Check sheet for the modelled part. Datum: model origin and axes. Units: mm. Face numbers are marked on the shaded views. Round coordinates to 2 decimals unless told otherwise and drop trailing zeros. Loops run counter-clockwise (first coordinate to the right, second up) from the corner with the lowest first, then second, coordinate; pieces in that order, holes last. Notation, with made-up numbers: (-5, 57) - (34, 57) arc R31 cw to (34, 87) - close; hole circle Ø6 at (-3.75, -15). An arc over 180 degrees is marked (long way). Put each result on its own line as item: value. Start each with the question number.
Item 1: Material ranges on line 1 along Z through (x, y) = (18.5, 6.5); line 2 along X through (y, z) = (15.5, 7); line 3 along Z through (x, y) = (-17, 7), recorded low to high.
Item 2: Draft check along Z on the marked faces 1, 2 and 3. Enter one of: pulls with the +Z half, pulls with the -Z half, needs draft (parallel to the pull), parting line crosses it, or undercut.
Item 3: Section check B-B, the plane y = 19.5. Record the cut outline in (x, z), and give its area (3 significant figures).
Item 4: Section check C-C, the plane y = 10. Record the cut outline in (x, z).
Item 5: Section check D-D, the plane z = 14.75. Record the cut outline in (x, y).
Item 6: Section check A-A, the plane z = 6.35. Record the cut outline in (x, y), and give its area (3 significant figures).
from build123d import *

# Parameters (mm, degrees)
PAD_DEPTH    = 25.4
SKETCH001_R  = 2.248154
POCKET_DEPTH = 30.2016


with BuildPart() as part:
    # Sketch → Pad (new body)
    with BuildSketch(Plane.XY):
        with BuildLine():
            ThreePointArc((11.935765, 0.8128), (0, 11.963408), (-11.935765, 0.8128))
            Line((-24.6634, 0.8128), (-11.935765, 0.8128))
            Line((-24.6634, 31.0134), (-24.6634, 0.8128))
            Line((-24.6634, 31.0134), (24.6634, 31.0134))
            Line((24.6634, 31.0134), (24.6634, 0.8128))
            Line((11.935765, 0.8128), (24.6634, 0.8128))
        make_face()
    extrude(amount=PAD_DEPTH)

    # Sketch001 (on Face4 of Pad) → Pocket (cut, through all)
    with BuildSketch(Plane(origin=(0, 31.0134, 0), x_dir=(-1, 0, 0), z_dir=(0, 1, 0))):
        with Locations((18.3134, 6.35)):
            Circle(SKETCH001_R)
        with Locations((18.3134, 19.05)):
            Circle(SKETCH001_R)
        with Locations((-18.3134, 19.05)):
            Circle(SKETCH001_R)
        with Locations((-18.3134, 6.35)):
            Circle(SKETCH001_R)
    extrude(amount=-POCKET_DEPTH, mode=Mode.SUBTRACT)


solid = part.part
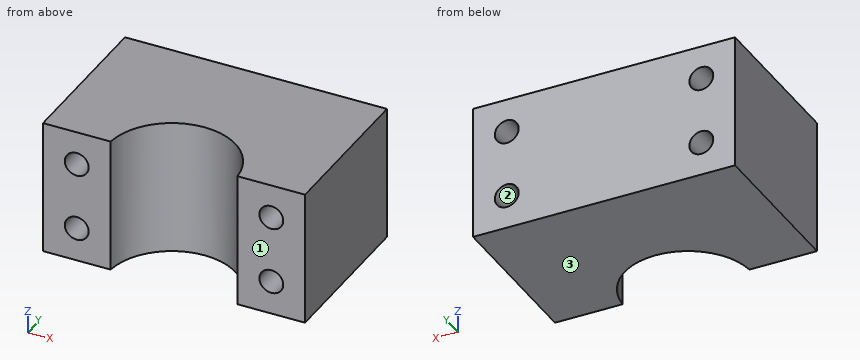
Check result:
1. line 1: 0 to 4.11, 8.59 to 16.81, 21.29 to 25.4
1. line 2: -24.66 to -20.47, -16.16 to 16.16, 20.47 to 24.66
1. line 3: 0 to 4.53, 8.17 to 17.23, 20.87 to 25.4
2. face 1: needs draft
2. face 2: undercut
2. face 3: pulls with the -Z half
3. outline: (-24.66, 0) - (24.66, 0) - (24.66, 25.4) - (-24.66, 25.4) - close; hole circle Ø4.5 at (-18.31, 6.35); hole circle Ø4.5 at (-18.31, 19.05); hole circle Ø4.5 at (18.31, 6.35); hole circle Ø4.5 at (18.31, 19.05)
3. area: 1,190 mm²
4. outline: (-24.66, 0) - (-6.57, 0) - (-6.57, 25.4) - (-24.66, 25.4) - close; (6.57, 0) - (24.66, 0) - (24.66, 25.4) - (6.57, 25.4) - close; hole circle Ø4.5 at (-18.31, 6.35); hole circle Ø4.5 at (-18.31, 19.05); hole circle Ø4.5 at (18.31, 6.35); hole circle Ø4.5 at (18.31, 19.05)
5. outline: (-24.66, 0.81) - (-11.94, 0.81) arc R11.96 cw to (11.94, 0.81) - (24.66, 0.81) - (24.66, 31.01) - (-24.66, 31.01) - close
6. outline: (-24.66, 0.81) - (-20.56, 0.81) - (-20.56, 31.01) - (-24.66, 31.01) - close; (-16.07, 0.81) - (-11.94, 0.81) arc R11.96 cw to (11.94, 0.81) - (16.07, 0.81) - (16.07, 31.01) - (-16.07, 31.01) - close; (20.56, 0.81) - (24.66, 0.81) - (24.66, 31.01) - (20.56, 31.01) - close
6. area: 1,010 mm²
